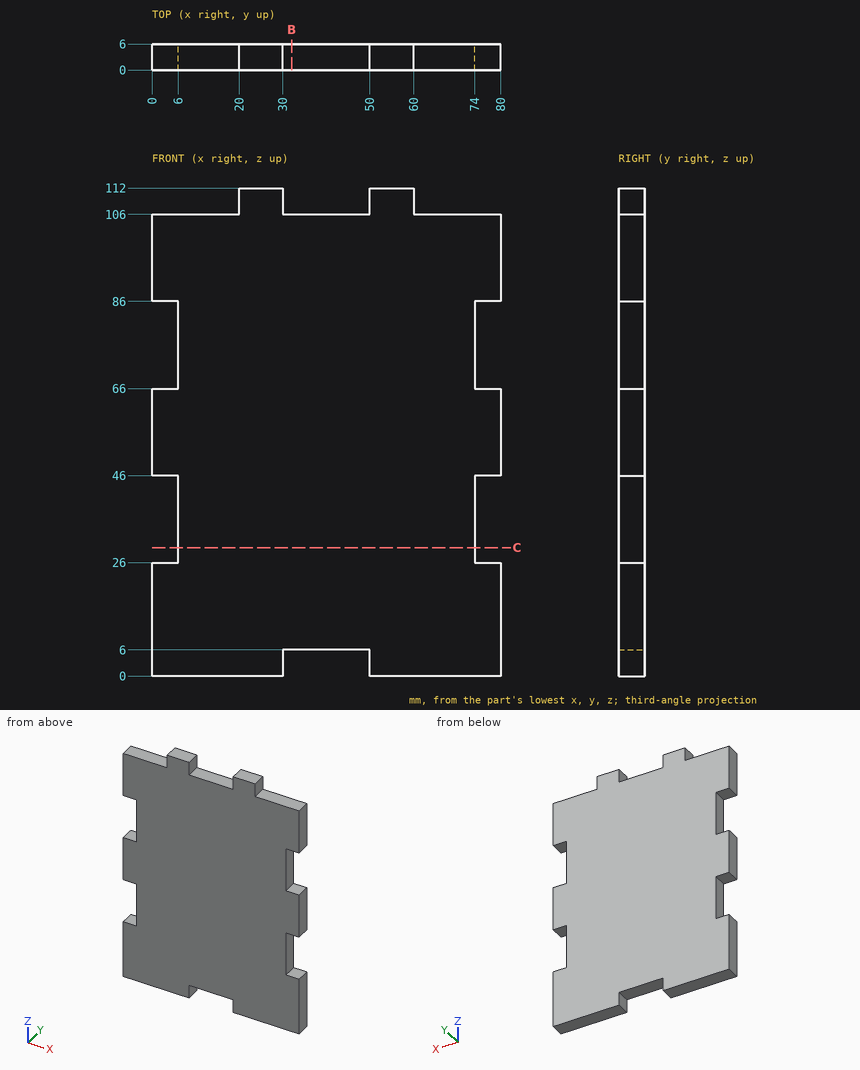
For this review, use the dimensioned drawing (mm, ordinates from the lowest corner) and the shaded views. Round coordinates to 2 decimals unless told otherwise and drop trailing zeros. Order: outer loops, then holes, each group sorted by start corner. A loop starts at its lowest first (then second) coordinate and runs counter-clockwise, first axis right, second up. Notation, with made-up numbers: (68, -37) -> (87, -37) arc R18 cw to (87, -11) -> close; hole circle Ø11 at (-14, 77). An arc over 180 degrees is marked (long way). One line per item, written item: value. Start each with the question number.
Q1. Wall thickness on line 1 (X direction, y = 4.8, z = 44.5); line 2 (Z direction, x = 48, y = 1.7); line 3 (Z direction, x = 12, y = 2.45): over which ranges is each line inside the solid? List them lowest first.
Q2. Take a section at C-C (z = 29.5). Write out the cut boundary in (x, y).
Q3. Take a section at B-B (x = 32). Write out the cut boundary in (y, z), and give its area (3 significant figures).
Q4. Clearance check with flat-ended pins moving along their axes: pin 1 Ø1.8 at (y, z) = (3, 110) entering from +X; pin 2 Ø3 at (y, z) = (3, 40) entering from -X; pin 3 Ø2 at (y, z) = (2.5, 29) entering from +X. State where each tip first meets the part, or that it passes through.
Reported:
1. line 1: x = 6 to 74
1. line 2: z = 6 to 106
1. line 3: z = 0 to 106
2. outline: (6, 0) -> (74, 0) -> (74, 6) -> (6, 6) -> close
3. outline: (0, 6) -> (6, 6) -> (6, 106) -> (0, 106) -> close
3. area: 600 mm2
4. pin 1: stops at x = 60
4. pin 2: stops at x = 6
4. pin 3: stops at x = 74
